```python
from build123d import *

# Parameters (mm, degrees)
SKETCH_1_R          = 31
SKETCH_1_R_2        = 15
EXTRUDE_1_DEPTH     = 16
SKETCH_2_R          = 27
SKETCH_2_R_2        = 22
CUT_EXTRUDE_1_DEPTH = 0.5
CUT_EXTRUDE_START   = -0.5
SKETCH_3_R          = 27
SKETCH_3_R_2        = 22
CUT_EXTRUDE_2_DEPTH = 0.5
SKETCH_4_R          = 19
SKETCH_4_R_2        = 17
CUT_EXTRUDE_3_DEPTH = 0.2
FILLET_1_R          = 0.5
CUT_EXTRUDE_START_2 = -0.2
SKETCH_5_R          = 19
SKETCH_5_R_2        = 17
CUT_EXTRUDE_4_DEPTH = 0.2


with BuildPart() as part:
    # 草图1 → 凸台-拉伸1 (new body)
    with BuildSketch(Plane.XY):
        Circle(SKETCH_1_R)
        Circle(SKETCH_1_R_2, mode=Mode.SUBTRACT)
    extrude(amount=EXTRUDE_1_DEPTH)

    # 草图2 → 切除-拉伸1 (cut)
    with BuildSketch(Plane.XY.offset(16)):
        Circle(SKETCH_2_R)
        Circle(SKETCH_2_R_2, mode=Mode.SUBTRACT)
    extrude(amount=-CUT_EXTRUDE_1_DEPTH, mode=Mode.SUBTRACT)

    # 草图3 → 切除-拉伸2 (cut)
    with BuildSketch(Plane(origin=(0, 0, 0), x_dir=(-1, 0, 0), z_dir=(0, 0, -1)).offset(CUT_EXTRUDE_START)):
        with Locations(Location((0, 0, 0), (0, 0, 180))):
            Circle(SKETCH_3_R)
        with Locations(Location((0, 0, 0), (0, 0, 180))):
            Circle(SKETCH_3_R_2, mode=Mode.SUBTRACT)
    extrude(amount=CUT_EXTRUDE_2_DEPTH, mode=Mode.SUBTRACT)

    # 草图4 → 切除-拉伸3 (cut)
    with BuildSketch(Plane.XY.offset(16)):
        Circle(SKETCH_4_R)
        Circle(SKETCH_4_R_2, mode=Mode.SUBTRACT)
    extrude(amount=-CUT_EXTRUDE_3_DEPTH, mode=Mode.SUBTRACT)

    # 圆角1
    fillet_1_edges = [part.edges().sort_by_distance(p)[0] for p in [
        (-22, 0, 16),
        (-22, 0, 0),
    ]]
    fillet(fillet_1_edges, radius=FILLET_1_R - 0.0001)  # a hair under: the kernel refuses the full size

    # 草图5 → 切除-拉伸4 (cut)
    with BuildSketch(Plane(origin=(0, 0, 0), x_dir=(-1, 0, 0), z_dir=(0, 0, -1)).offset(CUT_EXTRUDE_START_2)):
        with Locations(Location((0, 0, 0), (0, 0, 180))):
            Circle(SKETCH_5_R)
        with Locations(Location((0, 0, 0), (0, 0, 180))):
            Circle(SKETCH_5_R_2, mode=Mode.SUBTRACT)
    extrude(amount=CUT_EXTRUDE_4_DEPTH, mode=Mode.SUBTRACT)


solid = part.part
```
Here's how the part is built. I have some questions about the finished solid (model axes, mm). A direction names the side the tool comes from. Coordinates: 2 decimals unless noted, no trailing zeros. Loops run counter-clockwise (first coordinate to the right, second up) from the corner with the lowest first, then second, coordinate; pieces in that order, holes last. Notation, with made-up numbers: (72.5, -17) -> (114.5, -17) arc R23 ccw to (114.5, 7) -> close; hole circle Ø9 at (-8.5, -5). An arc over 180 degrees is marked (long way). Return JSON: item names as keys, results as strings.
1) For faces 4 (the face through (6, -14, 16)), 5 (the face through (-14, -10, 15.8)), 6 (the face through (-10, 20, 0.5)), which set-ups out of +Z, -Z, +X, -X, +Y, -Y let a thin tool reach every point of the face, with its end or its side?
Results below:
{"face 4": "+Z, +X, -X, +Y, -Y", "face 5": "+Z", "face 6": "-Z"}
2) Will these pins go through, and if not, where does the flat tip stop? pin 1 (1 mm diameter, centred on x = 17, z = 5, fed in from -Y); pin 2 (4 mm diameter, centred on x = 21.5, z = 4, fed in from +Y); pin 3 (2 mm diameter, centred on x = -6, z = 9, fed in from +Y).
Results below:
{"pin 1": "y = -26.24", "pin 2": "y = 24.1", "pin 3": "y = 30.59"}
3) If we section it at A-A, the plane z = 5.25: Write out the boundary of the cut face in (x, y).
Results below:
{"outline": "circle Ø62 at (0, 0); hole circle Ø30 at (0, 0)"}
4) Thinking about a two-plate mould opening in X: for faces 1 (the face through (-5.85, -26.36, 15.75)), 2 (the face through (6, -14, 0)), 3 (the face through (-4.036, 30.736, 7.888)), which applies, +X half, -X half, draft (parallel to the pull), parting line (faces both ways), or undercut?
Results below:
{"face 1": "undercut", "face 2": "draft", "face 3": "parting line"}
5) I need wall thicknesses on line 1 (Y direction, x = 0, z = 0.15); line 2 (Y direction, x = 0, z = 15.9); line 3 (Y direction, x = 0, z = 14.75). Which ranges of each line are inside material? Lowest first, please. Write a range as from..to.
Results below:
{"line 1": "-31..-27, -21.86..-19, -17..-15, 15..17, 19..21.86, 27..31", "line 2": "-31..-27, -21.8..-19, -17..-15, 15..17, 19..21.8, 27..31", "line 3": "-31..-15, 15..31"}
